Autodesk Inventor part; units mm, degrees
ref_plane "YZ Plane" through (0, 0, 0) normal (1, 0, 0) x (0, 1, 0)
ref_plane "XZ Plane" through (0, 0, 0) normal (0, 1, 0) x (-1, 0, 0)
ref_plane "XY Plane" through (0, 0, 0) normal (0, 0, 1) x (1, 0, 0)
sketch "Sketch1" plane through (0, 0, 0) normal (0, 0, 1) x (1, 0, 0)
  line L0 (21, -21) -> (-21, -21)
  line L1 (-21, -21) -> (-21, 21)
  line L2 (-21, 21) -> (21, 21)
  line L3 (21, 21) -> (21, -21)
  line L4 (21, -21) -> (-21, 21) construction
  line L5 (-21, -21) -> (21, 21) construction
  circle A0 centre (-15.5, 15.5) radius 1.5
  circle A1 centre (15.5, 15.5) radius 1.5
  circle A2 centre (15.5, -15.5) radius 1.5
  circle A3 centre (-15.5, -15.5) radius 1.5
  line L6 (-15.5, 15.5) -> (-15.5, -15.5) construction
  line L7 (-15.5, 15.5) -> (15.5, 15.5) construction
  line L8 (15.5, 15.5) -> (15.5, -15.5) construction
  circle A4 centre (-15.5, 15.5) radius 4.5
  circle A5 centre (15.5, 15.5) radius 4.5
  circle A6 centre (15.5, -15.5) radius 4.5
  circle A7 centre (-15.5, -15.5) radius 4.5
  circle A8 centre (0, 0) radius 10
  dimension "d0" = 42
  dimension "d1" = 42
  dimension "d2" = 31
  dimension "d3" = 3
  dimension "d4" = 3
  dimension "d7" = 20
extrude "Extrusion1" add sketch "Sketch1" along normal blind 8 contours L0 L1 L2 L3 | A4 | A5 | A6 | A7
sketch "Sketch2" plane through (0, 0, 8) normal (0, 0, 1) x (1, 0, 0)
  line L0 (21, 21) -> (-21, 21)
  line L1 (-21, 21) -> (-21, -21)
  line L2 (-21, -21) -> (21, -21)
  line L3 (21, -21) -> (21, 21)
  circle A0 centre (-15.5, 15.5) radius 1.5
  circle A1 centre (15.5, 15.5) radius 1.5
  circle A2 centre (15.5, -15.5) radius 1.5
  circle A3 centre (0, 0) radius 10
  circle A4 centre (-15.5, -15.5) radius 1.5
  circle A5 centre (-15.5, 15.5) radius 3.5
  circle A6 centre (15.5, 15.5) radius 3.5
  circle A7 centre (15.5, -15.5) radius 3.5
  circle A8 centre (-15.5, -15.5) radius 3.5
  dimension "d10" = 7
extrude "Extrusion3" cut sketch "Sketch2" against normal blind 5 contours A5 | A6 | A7 | A8
sketch "Sketch3" plane through (0, 0, 8) normal (0, 0, 1) x (1, 0, 0)
  circle A0 centre (15.5, -15.5) radius 3.5
  circle A1 centre (15.5, 15.5) radius 3.5
  circle A2 centre (-15.5, -15.5) radius 3.5
  circle A3 centre (-15.5, 15.5) radius 3.5
  line L0 (21, 21) -> (-21, 21)
  line L1 (-21, 21) -> (-21, -21)
  line L2 (-21, -21) -> (21, -21)
  line L3 (21, -21) -> (21, 21)
  circle A4 centre (0, 0) radius 10
  line L4 (-11, 21) -> (-11, -21)
  line L5 (-11, 11) -> (-1, 11)
  line L6 (-1, 11) -> (-1, 21)
  line L7 (-11, -11) -> (-1, -11)
  line L8 (-1, -11) -> (-1, -21)
  dimension "d13" = 10
  dimension "d14" = 10
  dimension "d15" = 10
extrude "Extrusion4" add sketch "Sketch3" along normal blind 10 contours L6 L5 L4 L0 | L2 L4 L7 L8
sketch "Sketch4" plane through (0, 0, 0) normal (0, 0, -1) x (-1, 0, 0)
  line L0 (21, 21) -> (21, -21)
  line L1 (21, 21) -> (41, 21)
  line L2 (41, 21) -> (41, -21)
  line L3 (41, -21) -> (21, -21)
  circle A0 centre (31, 15.5) radius 1.5
  circle A1 centre (31, -15.5) radius 1.5
  line L4 (31, 15.5) -> (31, -15.5) construction
  line L5 (31, 0) -> (21, 0) construction
  circle A2 centre (31, 0) radius 1.5
  point P0 (0, 0)
  dimension "d18" = 31
  dimension "d19" = 10
  dimension "d20" = 10
  dimension "d21" = 3
extrude "Extrusion5" add sketch "Sketch4" against normal up to surface (8 mm away)
sketch "Sketch5" plane through (-11, 11, 8) normal (-1, 0, 0) x (0, 0, 1)
  line L0 (0, 0) -> (0, 10)
  line L1 (0, 0) -> (10, 0)
  line L2 (10, 10) -> (10, 0)
  line L3 (0, 10) -> (10, 10)
  line L4 (0, -32) -> (0, -22)
  line L5 (0, -32) -> (10, -32)
  line L6 (10, -22) -> (10, -32)
  line L7 (0, -22) -> (10, -22)
  line L8 (10, 10) -> (0, 0) construction
  line L9 (10, 0) -> (0, 10) construction
  line L10 (10, -32) -> (0, -22) construction
  line L11 (10, -22) -> (0, -32) construction
  circle A0 centre (5, 5) radius 1.5
  circle A1 centre (5, -27) radius 1.5
  point P0 (-8, -11)
  dimension "d24" = 3
  dimension "d25" = 3
extrude "Extrusion6" cut sketch "Sketch5" against normal through all contours A0 | A1
draft "FaceDraft1" angle 45 pull direction (1, 0, 0) faces at (-7.6667, -14.3333, 18) (-7.6667, 17.6667, 18) fixed edges at (-1, -16, 18) (-1, 16, 18)
properties part number "end motor holder"
Source: CAD feature listing. Evaluate the final solid. Frame: model axes, mm. A direction names the side the tool comes from. Coordinates: 2 decimals unless noted, no trailing zeros. Write each loop counter-clockwise with the first axis right and the second up, starting at its lowest first coordinate (ties: lowest second). Pieces come first, ordered by that corner, then holes. Notation, with made-up numbers: (79, 30) -> (131, 30) arc R31 ccw to (131, 67) -> close; hole circle Ø2 at (-15.5, 35.25). An arc over 180 degrees is marked (long way). Return JSON: item names as keys, results as strings. Group by question number.
1) Section query B-B, the plane z = 20. Return loops of the section in (x, y), plus the area to 3 significant figures.
2) Set-up query: faces 4 (the face through (-11, -16, 18)), 5 (the face through (-1, -14.8, 11.8)), 6 (the face through (-6.07, 16.07, 11.5)), 7 (the face through (18.84, 16.55, 5.54)), 8 (the face through (-6, -11, 16)). Return all of +Z, -Z, +X, -X, +Y, -Y with unobstructed straight access to the full face (end or side cutting, diameter ignored); none if empty.
3) Contact query for flat-ended pins moving along their axis: P1, Ø9, axis at x = 15.5, y = -15.5, coming from the +Z side; P2, Ø2.5, axis at x = 15.5, y = -15.5, coming from the -Z side; P3, Ø2, axis at x = -16, y = -14, coming from the +Z side; P4, Ø11, axis at y = 15.5, z = 15, coming from the +X side. Output: stop coordinate, or through.
4) Section query C-C, the plane y = -8. Return loops of the section in (x, z), plus the area to 3 significant figures.
5) Ray query, line 1 along Y through (x, z) = (-15.5, 2.2); line 2 along X through (y, z) = (1, 7.5); line 3 along Z through (x, y) = (-20, -2). Return the intervals inside material, ascending.
6) Section query A-A, the plane x = -8. Return loops of the section in (y, z), plus the area to 3 significant figures.
7) Mould query, pull axis Z, two halves, no side actions, for faces 1 (the face through (-14.8, -17, 3)), 2 (the face through (-6.07, -15.93, 11.5)), 3 (the face through (-17, -15.57, 1.48)). Classes: +Z half, -Z half, draft (parallel to the pull), parting line (faces both ways), or undercut.
8) Section query D-D, the plane x = -31. Return loops of the section in (y, z).
From the geometry:
{
 "1": {"outline": "(-11, -21) -> (-3, -21) -> (-3, -11) -> (-11, -11) -> close; (-11, 11) -> (-3, 11) -> (-3, 21) -> (-11, 21) -> close", "area": "160 mm²"},
 "2": {"face 4": "+Z, -X, +Y, -Y", "face 5": "+Z, +X, +Y, -Y", "face 6": "+X, -X", "face 7": "+Z", "face 8": "+Z, +X, -X"},
 "3": {"P1": "z = 8", "P2": "through", "P3": "z = 3", "P4": "x = -1"},
 "4": {"outline": "(-41, 0) -> (-6, 0) -> (-6, 8) -> (-41, 8) -> close; (6, 0) -> (21, 0) -> (21, 8) -> (6, 8) -> close", "area": "400 mm²"},
 "5": {"line 1": "-21 to -17, -14 to 14, 17 to 21", "line 2": "-41 to -32.12, -29.88 to -9.95, 9.95 to 21", "line 3": "0 to 8"},
 "6": {"outline": "(-21, 0) -> (-6, 0) -> (-6, 8) -> (-11, 8) -> (-11, 25) -> (-21, 25) -> close; (6, 0) -> (21, 0) -> (21, 25) -> (11, 25) -> (11, 8) -> (6, 8) -> close; hole circle Ø3 at (-16, 13); hole circle Ø3 at (16, 13)", "area": "566 mm²"},
 "7": {"face 1": "+Z half", "face 2": "undercut", "face 3": "draft"},
 "8": {"outline": "(-21, 0) -> (-17, 0) -> (-17, 8) -> (-21, 8) -> close; (-14, 0) -> (-1.5, 0) -> (-1.5, 8) -> (-14, 8) -> close; (1.5, 0) -> (14, 0) -> (14, 8) -> (1.5, 8) -> close; (17, 0) -> (21, 0) -> (21, 8) -> (17, 8) -> close"}
}
